Here's how the part is built. I have some questions about the finished solid (model axes, mm). Give positions to 0.01 mm unless a question says otherwise; leave off trailing zeros. Loops run counter-clockwise (first coordinate to the right, second up) from the corner with the lowest first, then second, coordinate; pieces in that order, holes last. Notation, with made-up numbers: (-18.75, 68.25) - (-12.75, 68.25) arc R27 cw to (-12.75, 104.25) - close; hole circle Ø3 at (69, 78). An arc over 180 degrees is marked (long way). Use a Markdown table: item, result.
from build123d import *

# Parameters (mm, degrees)
SKETCH1_W           = 270
SKETCH1_H           = 20
BOSS_EXTRUDE1_DEPTH = 5
SKETCH2_W           = 5
SKETCH2_H           = 20
BOSS_EXTRUDE2_DEPTH = 19
SKETCH3_R           = 2
CUT_EXTRUDE1_DEPTH  = 272.248963132
SKETCH4_W           = 5
SKETCH4_H           = 5
BOSS_EXTRUDE3_DEPTH = 5
CUT_EXTRUDE2_DEPTH  = 139.567672998
SKETCH6_R           = 2
CUT_EXTRUDE3_DEPTH  = 138.480907765
SKETCH7_R           = 3.68294157
CUT_EXTRUDE4_DEPTH  = 10


with BuildPart() as part:
    # Sketch1 → Boss-Extrude1 (new body)
    with BuildSketch(Plane.XY):
        Rectangle(SKETCH1_W, SKETCH1_H)
    extrude(amount=BOSS_EXTRUDE1_DEPTH)

    # Sketch2 → Boss-Extrude2 (add)
    with BuildSketch(Plane.XY.offset(5)):
        with Locations((132.5, 0)):
            Rectangle(SKETCH2_W, SKETCH2_H)
    extrude(amount=BOSS_EXTRUDE2_DEPTH)

    # Sketch3 → Cut-Extrude1 (cut, through all)
    with BuildSketch(Plane(origin=(135, 0, 0), x_dir=(0, 0, -1), z_dir=(1, 0, 0))):
        with Locations((-14.5, 0)):
            Circle(SKETCH3_R)
    extrude(amount=-CUT_EXTRUDE1_DEPTH, mode=Mode.SUBTRACT)

    # Sketch4 → Boss-Extrude3 (add)
    with BuildSketch(Plane.ZY.offset(-130)):
        with Locations((7.5, -7.5)):
            Rectangle(SKETCH4_W, SKETCH4_H)
        with Locations((7.5, 7.5)):
            Rectangle(SKETCH4_W, SKETCH4_H)
    extrude(amount=BOSS_EXTRUDE3_DEPTH)

    # Sketch5 → Cut-Extrude2 (cut, through all)
    with BuildSketch(Plane.XZ.offset(10)):
        Polygon((125, 5), (130, 10), (125, 10), align=None)
    extrude(amount=-CUT_EXTRUDE2_DEPTH, mode=Mode.SUBTRACT)

    # Sketch6 → Cut-Extrude3 (cut, through all)
    with BuildSketch(Plane(origin=(0, 0, 0), x_dir=(-1, 0, 0), z_dir=(0, 0, -1))):
        with Locations((123, 0)):
            Circle(SKETCH6_R)
    extrude(amount=-CUT_EXTRUDE3_DEPTH, mode=Mode.SUBTRACT)

    # Sketch7 → Cut-Extrude4 (cut)
    with BuildSketch(Plane(origin=(0, 0, 0), x_dir=(-1, 0, 0), z_dir=(0, 0, -1))):
        Circle(SKETCH7_R)
    extrude(amount=-CUT_EXTRUDE4_DEPTH, mode=Mode.SUBTRACT)


solid = part.part
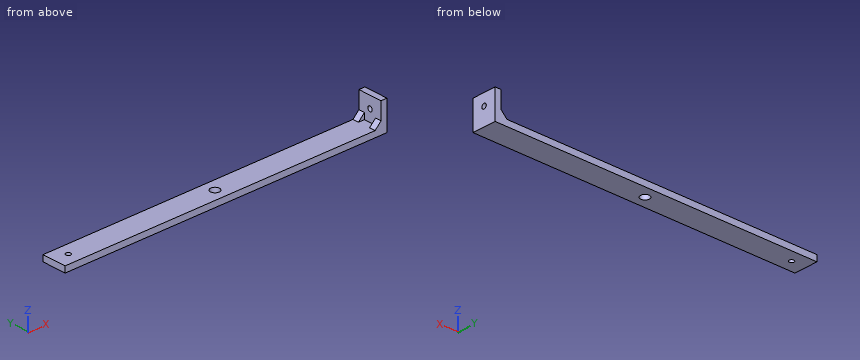
(1) Will these pins go through, and if not, where does the flat tip stop? pin 1 (10 mm diameter, centred on x = -19.5, y = 4.5, fed in from +Z); pin 2 (9.5 mm diameter, centred on y = -3.5, z = 19, fed in from -X).
A:
| item | result |
|---|---|
| pin 1 | z = 5 |
| pin 2 | x = 130 |
(2) Suppose I cut it at B-B on x = -89.5. Write out the boundary of the cut face in (y, z), plus the area to 3 significant figures.
A:
| item | result |
|---|---|
| outline | (-10, 0) - (10, 0) - (10, 5) - (-10, 5) - close |
| area | 100 mm2 |
(3) If I drill on line 1 (Y direction, x = -123, z = 2.05); line 2 (Y direction, x = 0, z = 2.3); line 3 (X direction, y = -7.5, z = 17), over which ranges is the centre line in solid material (lowest first)?
A:
| item | result |
|---|---|
| line 1 | -10 to -2, 2 to 10 |
| line 2 | -10 to -3.68, 3.68 to 10 |
| line 3 | 130 to 135 |
(4) Suppose I cut it at A-A on x = 0. Write out the boundary of the cut face in (y, z).
A:
| item | result |
|---|---|
| outline | (-10, 0) - (-3.68, 0) - (-3.68, 5) - (-10, 5) - close; (3.68, 0) - (10, 0) - (10, 5) - (3.68, 5) - close |
(5) Suppose I cut it at C-C on z = 20.25. Write out the boundary of the cut face in (x, y).
A:
| item | result |
|---|---|
| outline | (130, -10) - (135, -10) - (135, 10) - (130, 10) - close |
